Read the model definition and answer for the solid it produces. Units are mm, in the model's axes. Face numbers are marked on the shaded views. A direction names the side the tool comes from. Round coordinates to 2 decimals unless told otherwise and drop trailing zeros. Write each loop counter-clockwise with the first axis right and the second up, starting at its lowest first coordinate (ties: lowest second). Pieces come first, ordered by that corner, then holes. Notation, with made-up numbers: (-21, -17) - (-13, -17) arc R25 cw to (-13, 12) - close; hole circle Ø1 at (30.5, -10). An arc over 180 degrees is marked (long way). Answer as CSV lines item,"result". Start each with the question number.
1) For a pull along X with two mould halves and no side action, classify the marked faces 3, 4, 5 and 6 as +X half, -X half, draft (parallel to the pull), parting line (faces both ways), or undercut.
2) Find section C-C on z = -10. Determine the outline of the cut face in (x, y).
3) Find section B-B on y = 7.5. Determine the outline of the cut face in (x, z).
4) Find section D-D on x = 45. Determine the outline of the cut face in (y, z).
5) Each of these flat-tipped pins is pushed along its axis until it touches: pin 1 (20 mm diameter, centred on x = 67, y = 27.5, fed in from +Z); pin 2 (6 mm diameter, centred on x = 30, y = 34.5, fed in from -Z); pin 3 (2 mm diameter, centred on y = 35, z = -10, fed in from +X). Where does it stop, or does it pass through?
6) Consider line 1 along X through (y, z) = (6.5, -13.5); line 2 along Y through (x, z) = (104.25, -10); line 3 along Z through (x, y) = (33.5, 32.5). Determine where each line is inside the solid, lowest interval first.
7) Find section A-A on z = -5. Determine the outline of the cut face in (x, y).
8) Which of the six approach directions +Z, -Z, +X, -X, +Y, -Y give full straight-line access (tool end or side, diameter ignored) to the marked faces 1 and 2?
from build123d import *

# Parameters (mm, degrees)
BODY_DEPTH   = 40
SKETCH2_R    = 8.5
SKETCH2_R_2  = 6
NOZZLE_DEPTH = 12


with BuildPart() as part:
    # Sketch1 → Body (new body)
    with BuildSketch(Plane(origin=(0, 0, 0), x_dir=(1, 0, 0), z_dir=(0, 1, 0))):
        Polygon((0, 0), (0, 20), (6, 20), (6, 13), (94, 13), (94, 20), (100, 20), (100, 0), (94, 0), (94, 7), (6, 7), (6, 0), align=None)
    extrude(amount=BODY_DEPTH)

    # Sketch2 → Nozzle (add)
    with BuildSketch(Plane(origin=(100, 0, 0), x_dir=(0, 0, -1), z_dir=(1, 0, 0))):
        with Locations((10, 20)):
            Circle(SKETCH2_R)
        with Locations((10, 20)):
            Circle(SKETCH2_R_2, mode=Mode.SUBTRACT)
    extrude(amount=NOZZLE_DEPTH)


solid = part.part
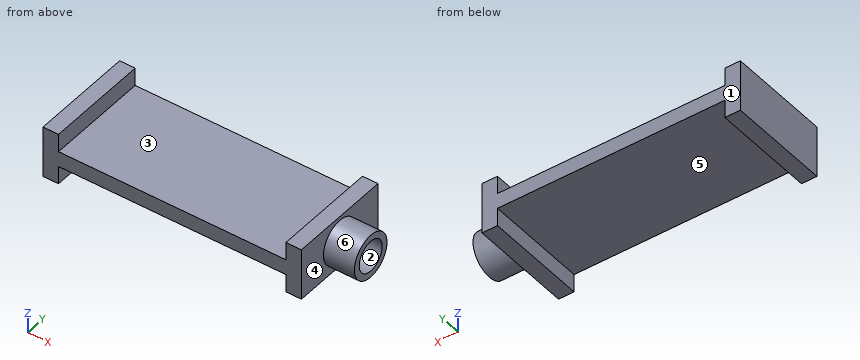
Check values:
1,face 3,"undercut"
1,face 4,"+X half"
1,face 5,"undercut"
1,face 6,"draft"
2,outline,"(0, 0) - (100, 0) - (100, 11.5) - (112, 11.5) - (112, 14) - (100, 14) - (100, 26) - (112, 26) - (112, 28.5) - (100, 28.5) - (100, 40) - (0, 40) - close"
3,outline,"(0, -20) - (6, -20) - (6, -13) - (94, -13) - (94, -20) - (100, -20) - (100, 0) - (94, 0) - (94, -7) - (6, -7) - (6, 0) - (0, 0) - close"
4,outline,"(0, -13) - (40, -13) - (40, -7) - (0, -7) - close"
5,pin 1,"stops at z = -7"
5,pin 2,"stops at z = -13"
5,pin 3,"stops at x = 100"
6,line 1,"x = 0 to 6, 94 to 100"
6,line 2,"y = 11.5 to 14, 26 to 28.5"
6,line 3,"z = -13 to -7"
7,outline,"(0, 0) - (6, 0) - (6, 40) - (0, 40) - close; (94, 0) - (100, 0) - (100, 13.13) - (112, 13.13) - (112, 16.68) - (100, 16.68) - (100, 23.32) - (112, 23.32) - (112, 26.87) - (100, 26.87) - (100, 40) - (94, 40) - close"
8,face 1,"+Z, -Z, +X, -X, +Y"
8,face 2,"+X"
